The drawing under review shows one solid part. Ordinate dimensions are in mm from its lowest x, y, z. A direction names the side the tool comes from. Coordinates: 2 decimals unless noted, no trailing zeros. Write each loop counter-clockwise with the first axis right and the second up, starting at its lowest first coordinate (ties: lowest second). Pieces come first, ordered by that corner, then holes.
1) We need section D-D on z = 8. Write out the cut boundary in (x, y).
2) For the marked faces 1 and 2, list the 3-axis set-ups (+Z, -Z, +X, -X, +Y, -Y) from which the entire face can be reached by the end or side of a thin tool; tool diameter is ignored.
3) Mouldability with a two-part tool opening along X and no side actions: class the marked faces 3 and 4 as pulls with the +X half, pulls with the -X half, needs draft (parallel to the pull), parting line crosses it, or undercut.
4) We need section B-B on z = 4.25. Write out the cut boundary in (x, y), then the cut area to 3 significant figures.
5) We need section A-A on y = 1.95. Write out the cut boundary in (x, z), then the cut area to 3 significant figures.
6) To check wall thickness, follow line 1 along X through (y, z) = (2, 5); line 2 along Z through (x, y) = (35, 1.7); line 3 along X through (y, z) = (0.9, 5). State the ranges of each line that lie inside material, in increasing order.
7) Insertion check: P1, Ø1, axis at x = 27, z = 3.5, coming from the +Y side. The pin has a flat end and moves straight along its axis. Give the tip position at first contact, or say it passes through.
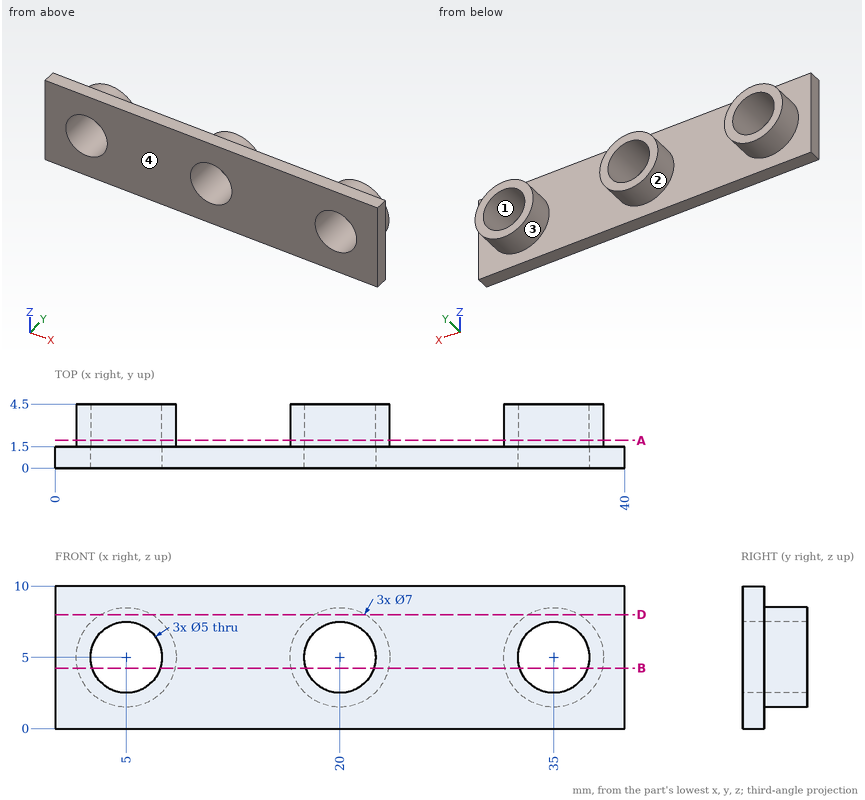
Result:
1. outline: (0, 0) - (40, 0) - (40, 1.5) - (36.8, 1.5) - (36.8, 4.5) - (33.2, 4.5) - (33.2, 1.5) - (21.8, 1.5) - (21.8, 4.5) - (18.2, 4.5) - (18.2, 1.5) - (6.8, 1.5) - (6.8, 4.5) - (3.2, 4.5) - (3.2, 1.5) - (0, 1.5) - close
2. face 1: +Y, -Y
2. face 2: +Y
3. face 3: undercut
3. face 4: needs draft
4. outline: (0, 0) - (2.62, 0) - (2.62, 4.5) - (1.58, 4.5) - (1.58, 1.5) - (0, 1.5) - close; (7.38, 0) - (17.62, 0) - (17.62, 4.5) - (16.58, 4.5) - (16.58, 1.5) - (8.42, 1.5) - (8.42, 4.5) - (7.38, 4.5) - close; (22.38, 0) - (32.62, 0) - (32.62, 4.5) - (31.58, 4.5) - (31.58, 1.5) - (23.42, 1.5) - (23.42, 4.5) - (22.38, 4.5) - close; (37.38, 0) - (40, 0) - (40, 1.5) - (38.42, 1.5) - (38.42, 4.5) - (37.38, 4.5) - close
4. area: 57.1 mm2
5. outline: circle Ø7 at (5, 5); circle Ø7 at (20, 5); circle Ø7 at (35, 5); hole circle Ø5 at (5, 5); hole circle Ø5 at (20, 5); hole circle Ø5 at (35, 5)
5. area: 56.5 mm2
6. line 1: x = 1.5 to 2.5, 7.5 to 8.5, 16.5 to 17.5, 22.5 to 23.5, 31.5 to 32.5, 37.5 to 38.5
6. line 2: z = 1.5 to 2.5, 7.5 to 8.5
6. line 3: x = 0 to 2.5, 7.5 to 17.5, 22.5 to 32.5, 37.5 to 40
7. P1: stops at y = 1.5
